from build123d import *

# Parameters (mm, degrees)
F1_R      = 51
F2_DEPTH  = 102
F4_W      = 285
F4_H      = 102
F4_R      = 75
F5_DEPTH  = 102
F9_R      = 38
F10_DEPTH = 75


# Not quite as in the source:
# - a pattern or mirror of a feature is missing from the dataset's text; its kind, count and spacing are read off the source's solid


with BuildPart() as f2:
    # F1 (on offset) → F2 (new body)
    with BuildSketch(Plane.XZ.offset(253)):
        with BuildLine():
            Line((0, -382.5), (0, 382.5))
            Line((0, 382.5), (-285, 382.5))
            Line((-285, 382.5), (-711.024961042, -137.4305074422))
            ThreePointArc((-711.024961042, -137.4305074422), (-730.5736402913, -296.6855751565), (-595, -382.5))
            Line((-595, -382.5), (0, -382.5))
        make_face()
        with Locations((-595, -232.5)):
            Circle(F1_R, mode=Mode.SUBTRACT)
    extrude(amount=F2_DEPTH)


with BuildPart() as f3_1:
    # F3: instance of F2
    add(f2.part.mirror(Plane.XZ))


with BuildPart() as f5:
    # F4 (on face) → F5 (new body)
    with BuildSketch(Plane.XY.offset(382.5)):
        with Locations((-142.5, -304)):
            Rectangle(F4_W, F4_H)
        with BuildLine():
            Line((311.2296497268, 178.2626096976), (0, 355))
            Line((0, 355), (-285, 355))
            Line((-285, 355), (-285, -253))
            Line((-285, -253), (0, -253))
            Line((0, -253), (0, -355))
            Line((0, -355), (311.2296497268, -178.2626096976))
            ThreePointArc((311.2296497268, -178.2626096976), (415, 0), (311.2296497268, 178.2626096976))
        make_face()
        with Locations((210, 0)):
            Circle(F4_R, mode=Mode.SUBTRACT)
    extrude(amount=-F5_DEPTH)


with BuildPart() as f6_1:
    # F6: instance of F5
    add(f5.part.mirror(Plane.XY))

    # F7: union F2, F3_1, F5
    add(f2.part)
    add(f3_1.part)
    add(f5.part)

    # F9 (on offset) → F10 (join)
    with BuildSketch(Plane.XZ.offset(100)):
        with BuildLine():
            Line((-234.9733120798, 382.5), (0, 382.5))
            Line((0, 382.5), (-220.5580805505, 645.3508848718))
            ThreePointArc((-220.5580805505, 645.3508848718), (-347.352965303, 656.4439998807), (-358.446080312, 529.6491151282))
            Line((-358.446080312, 529.6491151282), (-234.9733120798, 382.5))
        make_face()
        with Locations((-289.5020804312, 587.5)):
            Circle(F9_R, mode=Mode.SUBTRACT)
    f10 = extrude(amount=F10_DEPTH)

    # F10_copies: F10 across plane
    add(f10.mirror(Plane.ZX))


solid = f6_1.part
Input: part model. Units: mm. Frame: model coordinates. A direction names the side the tool comes from. Coordinates: 2 decimals unless noted, no trailing zeros. Loops run counter-clockwise (first coordinate to the right, second up) from the corner with the lowest first, then second, coordinate; pieces in that order, holes last. Notation, with made-up numbers: (11.25, 36) -> (62.25, 36) arc R26 ccw to (62.25, 75) -> close; hole circle Ø9 at (10, 44.5). An arc over 180 degrees is marked (long way). Write item = value, one per line. Start each with the question number.
Item 1: Material intervals for line 1 (Z direction, x = -168, y = -191); line 2 (Y direction, x = -545, z = -322.5); line 3 (X direction, y = 291, z = -232), sorted ascending.
Item 2: Cut plane D-D, the plane x = 98. Return loops of the section in (y, z), plus the area to 3 significant figures.
Item 3: Reachability of faces 4 (the face through (0, -303, -4)), 5 (the face through (-297.57, -136.98, 457.1)), 6 (the face through (-285, 4, -332)), 7 (the face through (-235, 175, 499)) from +Z, -Z, +X, -X, +Y, -Y: full face, straight path, thin tool, end or side. Return the list, or none.
Item 4: Cut plane B-B, the plane y = 0. Return loops of the section in (x, z), plus the area to 3 significant figures.
Item 5: Mould query, pull axis Y, two halves, no side actions, for faces 1 (the face through (-235, -175, 499)), 2 (the face through (-8, 5, 382.5)), 3 (the face through (-297.74, -136.975, 550.404)). Classes: pulls with the +Y half, pulls with the -Y half, needs draft (parallel to the pull), parting line crosses it, or undercut.
Item 6: First-contact query: P1, Ø10, axis at x = -51.5, y = -270.5, coming from the +Z side; P2, Ø1, axis at y = 264, z = 280.5, coming from the -X side. Flat tips, straight axial feed; report the tip coordinate or a pass-through.
Item 7: Cut plane C-C, the plane z = 454.5. Return loops of the section in (x, y), plus the area to 3 significant figures.
Item 8: Cut plane A-A, the plane z = -232.5. Return loops of the section in (x, y).
Ans:
q1.line_1 = -382.5 to -280.5, 280.5 to 382.5
q1.line_2 = -355 to -253, 253 to 355
q1.line_3 = -745 to -646, -544 to 0
q2.outline = (-299.35, -382.5) -> (299.35, -382.5) -> (299.35, -280.5) -> (-299.35, -280.5) -> close; (-299.35, 280.5) -> (299.35, 280.5) -> (299.35, 382.5) -> (-299.35, 382.5) -> close
q2.area = 122,000 mm²
q3.face_4 = +X, +Y, -Y
q3.face_5 = -X, +Y, -Y
q3.face_6 = -Z, -X
q3.face_7 = +Z, +X, -X, +Y
q4.outline = (-285, -382.5) -> (135, -382.5) -> (135, -280.5) -> (-285, -280.5) -> close; (-285, 280.5) -> (135, 280.5) -> (135, 382.5) -> (-285, 382.5) -> close; (285, -382.5) -> (415, -382.5) -> (415, -280.5) -> (285, -280.5) -> close; (285, 280.5) -> (415, 280.5) -> (415, 382.5) -> (285, 382.5) -> close
q4.area = 112,000 mm²
q5.face_1 = pulls with the -Y half
q5.face_2 = undercut
q5.face_3 = needs draft
q6.P1 = 382.5
q6.P2 = -368.99
q7.outline = (-295.39, -175) -> (-60.42, -175) -> (-60.42, -100) -> (-295.39, -100) -> close; (-295.39, 100) -> (-60.42, 100) -> (-60.42, 175) -> (-295.39, 175) -> close
q7.area = 35,200 mm²
q8.outline = (-745, -355) -> (-646, -355) -> (-646, -253) -> (-745, -253) -> close; (-745, 253) -> (-646, 253) -> (-646, 355) -> (-745, 355) -> close; (-544, -355) -> (0, -355) -> (0, -253) -> (-544, -253) -> close; (-544, 253) -> (0, 253) -> (0, 355) -> (-544, 355) -> close
